from build123d import *

# Parameters (mm, degrees)
SKETCH1_R           = 55
BOSS_EXTRUDE1_DEPTH = 20
BOSS_EXTRUDE1_TAPER = 10
SKETCH2_R           = 38.1
SKETCH2_R_2         = 35.55
CUT_EXTRUDE1_DEPTH  = 15
SKETCH3_R           = 51.473460386
SKETCH3_R_2         = 49.473460386
BOSS_EXTRUDE2_DEPTH = 2
BOSS_EXTRUDE2_TAPER = 10


with BuildPart() as part:
    # Sketch1 → Boss-Extrude1 (new body)
    with BuildSketch(Plane.XY):
        Circle(SKETCH1_R)
    extrude(amount=BOSS_EXTRUDE1_DEPTH, taper=BOSS_EXTRUDE1_TAPER)

    # Sketch2 → Cut-Extrude1 (cut)
    with BuildSketch(Plane.XY.offset(20)):
        Circle(SKETCH2_R)
        Circle(SKETCH2_R_2, mode=Mode.SUBTRACT)
    extrude(amount=-CUT_EXTRUDE1_DEPTH, mode=Mode.SUBTRACT)

    # Sketch3 → Boss-Extrude2 (add)
    with BuildSketch(Plane.XY.offset(20)):
        Circle(SKETCH3_R)
        Circle(SKETCH3_R_2, mode=Mode.SUBTRACT)
    extrude(amount=BOSS_EXTRUDE2_DEPTH, taper=BOSS_EXTRUDE2_TAPER)


solid = part.part
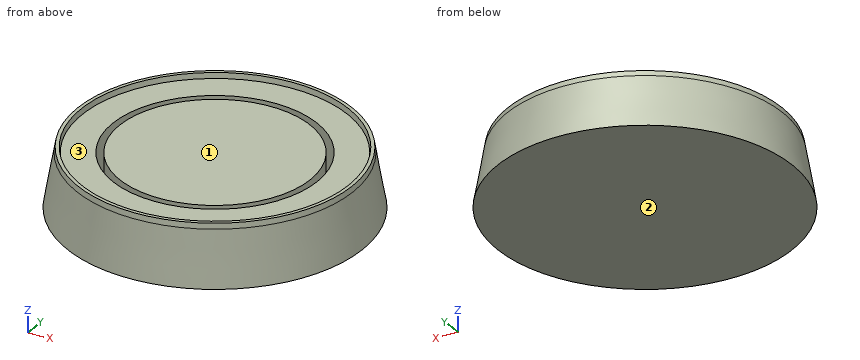
Design review of the part built by this model. Coordinates are the model's own, in mm. Face numbers are marked on the shaded views. Coordinates: 2 decimals unless noted, no trailing zeros. Order: outer loops, then holes, each group sorted by start corner. A loop starts at its lowest first (then second) coordinate and runs counter-clockwise, first axis right, second up. Notation, with made-up numbers: (39.5, -19.5) -> (96.5, -19.5) arc R20 ccw to (96.5, 19.5) -> close; hole circle Ø11 at (44, 22). An arc over 180 degrees is marked (long way). One line per item, written item: value.
1) We need section A-A, the plane z = 6.75. Give the boundary of the cut face in (x, y), then the cut area to 3 significant figures.
Output values:
outline: circle Ø107.62 at (0, 0); circle Ø71.1 at (0, 0); hole circle Ø76.2 at (0, 0)
area: 8,510 mm2
2) Draft analysis for pull direction X (two halves, no side actions). For the marked faces 1, 2 and 3, state which applies: +X half, -X half, draft (parallel to the pull), parting line (faces both ways), or undercut.
Output values:
face 1: undercut
face 2: draft
face 3: undercut
3) To check wall thickness, follow probe 1 along X at (y, z) = (-26, 11.75); probe 2 along Y at (x, z) = (-28, 6); probe 3 along X at (y, z) = (-5.5, 14.75). State the ranges of each line that lie inside material, in increasing order. Write a range as [from, to].
Output values:
probe 1: x = [-46.1, -27.85], [-24.24, 24.24], [27.85, 46.1]
probe 2: y = [-46.11, -25.84], [-21.9, 21.9], [25.84, 46.11]
probe 3: x = [-52.11, -37.7], [-35.12, 35.12], [37.7, 52.11]
4) Clearance check with flat-ended pins moving along their axes: P1, Ø3, axis at y = -12, z = 5.5, coming from the +X side; P2, Ø3, axis at y = 40, z = 14.5, coming from the -X side; P3, Ø4, axis at y = 32.5, z = 11.5, coming from the +X side. State where each tip first meets the part, or that it passes through.
Output values:
P1: stops at x = 53.1
P2: stops at x = -35.66
P3: stops at x = 43.38
